Autodesk Inventor part; units mm, degrees
ref_plane "Work Plane1" through (0, 4.572, 5.08) normal (0, 1, 0) x (-1, 0, 0)
ref_plane "YZ Plane" through (0, 0, 0) normal (1, 0, 0) x (0, 1, 0)
ref_plane "XY Plane" through (0, 0, 0) normal (0, 0, 1) x (1, 0, 0)
sketch "Sketch1" plane through (0, 0, 0) normal (0, 0, 1) x (1, 0, 0)
  circle A0 centre (0, 0) radius 21.59
  dimension "d0" = 43.18
extrude "Extrusion1" add sketch "Sketch1" along normal blind 5.08
sketch "Sketch2" plane through (0, 0, 5.08) normal (0, 0, 1) x (1, 0, 0)
  circle A0 centre (0, 0) radius 10.3632
  circle A1 centre (0, 0) radius 19.304
  dimension "d3" = 20.7264
  dimension "d4" = 38.608
extrude "Extrusion2" cut sketch "Sketch2" against normal blind 1.7272
sketch "Sketch3" plane through (0, 0, 5.08) normal (0, 0, 1) x (1, 0, 0)
  circle A0 centre (0, 0) radius 4.572
  dimension "d7" = 9.144
extrude "Extrusion3" add sketch "Sketch3" along normal blind 0.0025 and the other way blind 12.7
sketch "Sketch5" plane through (0, 0, 5.0825) normal (0, 0, 1) x (1, 0, 0)
  arc A0 (-1.2065, -1.0318) -> (-1.2065, 1.0318) centre (0, 0) ccw
  line L0 (-1.2065, -1.0318) -> (-1.2065, 1.0318)
extrude "Extrusion5" cut sketch "Sketch5" against normal blind 11.43
sketch "Sketch6" plane through (0, 0, 5.0825) normal (0, 0, 1) x (1, 0, 0)
  circle A0 centre (0, 0) radius 1.5875
  dimension "d19" = 3.175
extrude "Extrusion6" cut sketch "Sketch6" against normal blind 4.572
sketch "Sketch8" plane through (0, 0, 0) normal (0, 0, -1) x (-1, 0, 0)
  circle A0 centre (0, 0) radius 10.3632
  circle A1 centre (12.7, 0) radius 1.6891
  circle A2 centre (-12.7, 0) radius 1.6891
  circle A3 centre (0, 0) radius 4.572
  circle A4 centre (0, 0) radius 6.6294
  circle A5 centre (0, -12.7) radius 1.6891
  circle A6 centre (0, 12.7) radius 1.6891
  dimension "d25" = 3.3782
  dimension "d26" = 3.3782
  dimension "d29" = 3.3782
  dimension "d30" = 3.3782
  dimension "d38" = 12.7
  dimension "d39" = 12.7
  dimension "d40" = 12.7
  dimension "d41" = 12.7
extrude "Extrusion8" cut sketch "Sketch8" against normal blind 25.4 contours A1 | A2 | A5 | A6
ref_plane "Work Plane1" through (0, 4.572, 5.08) normal (0, 1, 0) x (-1, 0, 0)
sketch "Sketch9" plane through (0, 4.572, 5.08) normal (0, 1, 0) x (-1, 0, 0)
  circle A0 centre (0, -9.7924) radius 1.27
  point P0 (0, -5.08)
  dimension "d35" = 2.54
extrude "Extrusion9" cut sketch "Sketch9" against normal blind 25.4
properties part number "Shaft"
CAD build for the part. Positions are in the model's coordinates, mm. A direction names the side the tool comes from. Round coordinates to 2 decimals unless told otherwise and drop trailing zeros. Write each loop counter-clockwise with the first axis right and the second up, starting at its lowest first coordinate (ties: lowest second). Pieces come first, ordered by that corner, then holes. Notation, with made-up numbers: (78, 21.5) - (131, 21.5) arc R24 ccw to (131, 42.5) - close; hole circle Ø7 at (-25.75, 68.25). An arc over 180 degrees is marked (long way). Write item = value, one per line. Start each with the question number.
Q1. Band-saw the part on C-C (z = -2.25). Give the cut face in (x, y), then the cut area to 3 significant figures.
Q2. Drop flat-ended pins along their axis: pin 1 (5 mm diameter, centred on x = 4, y = 6.5, fed in from +Z); pin 2 (4 mm diameter, centred on x = -12.7, y = 0, fed in from +Z); pin 3 (2 mm diameter, centred on x = 0, y = -0.5, fed in from +Z); pin 4 (13 mm diameter, centred on x = 3, y = 5, fed in from -Z). Give the stop position or say it passes through.
Q3. Band-saw the part on A-A (x = 0). Count the separate pieces of the cut face and the enclosed holes in it, then the cut area to 3 significant figures.
Q4. Mould opens along X. For faces 1 (the flat face through (2, 0, 5.082)), 2 (the cylindrical face through (2.11, -4.056, -3.757)), 3 (the flat face through (0, 0, -6.348)) say: pulls with the +X half, pulls with the -X half, needs draft (parallel to the pull), parting line crosses it, or undercut.
Q5. Band-saw the part on B-B (y = -9). Give the cut face in (x, z).
Q6. Band-saw the part on D-D (x = -12.7). Give the cut face in (y, z).
Q7. Probe L1, parallel to Y at x = 0, z = 4.65; L2, parallel to Y at x = 0, z = -2.75; L3, parallel to X at y = 8.5, z = 3.5. List the from-to ranges inside material, lowest first. Write a range as from..to.
Q8. Which spindle directions (+Z, -Z, +X, -X, +Y, -Y) get a long thin tool onto all of the face, cutting with end or side? Do faces 4 (the cylindrical face through (-15.913, -14.592, 2.504)), 5 (the cylindrical face through (-1.587, 0.016, 2.829)). Say none if no direction does.
Answers below:
q1.outline = circle Ø9.14 at (0, 0); hole (-1.21, -1.03) arc R1.59 ccw (long way) to (-1.21, 1.03) - close
q1.area = 58.3 mm2
q2.pin_1 = 5.08
q2.pin_2 = 3.35
q2.pin_3 = -6.35
q2.pin_4 = -7.62
q3.separate_pieces = 5
q3.enclosed_holes = 0
q3.area = 184 mm2
q4.face_1 = needs draft
q4.face_2 = parting line crosses it
q4.face_3 = undercut
q5.outline = (-19.62, 0) - (19.62, 0) - (19.62, 5.08) - (17.08, 5.08) - (17.08, 3.35) - (5.14, 3.35) - (5.14, 5.08) - (-5.14, 5.08) - (-5.14, 3.35) - (-17.08, 3.35) - (-17.08, 5.08) - (-19.62, 5.08) - close
q6.outline = (-17.46, 0) - (-1.69, 0) - (-1.69, 3.35) - (-14.54, 3.35) - (-14.54, 5.08) - (-17.46, 5.08) - close; (1.69, 0) - (17.46, 0) - (17.46, 5.08) - (14.54, 5.08) - (14.54, 3.35) - (1.69, 3.35) - close
q7.L1 = -21.59..-19.3, -10.36..-1.59, 1.59..10.36, 19.3..21.59
q7.L2 = -4.57..-1.59, 1.59..4.57
q7.L3 = -19.85..-17.33, -5.93..5.93, 17.33..19.85
q8.face_4 = +Z, -Z
q8.face_5 = +Z
